Model file for the job. Use its own axes, mm. Give positions to 0.01 mm unless a question says otherwise; leave off trailing zeros. Loops run counter-clockwise (first coordinate to the right, second up) from the corner with the lowest first, then second, coordinate; pieces in that order, holes last. Notation, with made-up numbers: M 20.25,66.5 L 39.25,66.5 A7 ccw 39.25,79.5 Z; hole C -0.5,9 d5. An arc over 180 degrees is marked long. Use CSV: the item, a comma, the result in double quotes. Start each with the question number.
(1) Wall check: line 1 along X through (y, z) = (-0.05, 8.89) (3 decimals); line 2 along X through (y, z) = (2.5, 16.5); line 3 along Y through (x, z) = (-41.5, -7.5). Give the ranges that are in metal, low to high. Write a range as from..to.
(2) Slice it at A-A on x = 60.5. List the corners of the cut face in (y, z).
(3) Flat gauge pins, fed straight in: P1, Ø4, axis at x = 14.86, z = -7.65, coming from the -Y side; P2, Ø1.4, axis at y = 0.5, z = -6, coming from the +X side; P3, Ø3, axis at y = -0.5, z = 16, coming from the -X side; P4, Ø15, axis at x = -34.925, z = 8.89, coming from the -Y side. Where does each tip first touch, or does it go through?
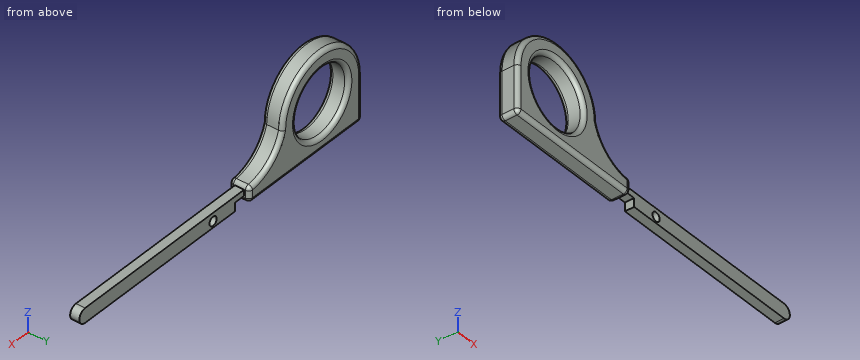
```python
from build123d import *

# Parameters (mm, degrees)
F0_R     = 12.7
F0_R_2   = 1.7145
F1_DEPTH = 1.778
F2_DEPTH = 3.81
F3_R     = 1.524


with BuildPart() as f1:
    # F0 (on Front) → F1 (new body, symmetric)
    with BuildSketch(Plane.XZ):
        with BuildLine():
            ThreePointArc((-15.875, 8.889999828), (-34.925, 27.939999828), (-53.975, 8.889999828))
            Line((-53.975, 8.889999828), (-53.975, -7.366000172))
            ThreePointArc((-53.975, -7.366000172), (-53.5286307345, -8.4436309065), (-52.451, -8.890000172))
            Line((-52.451, -8.890000172), (-1.5220896796, -8.890000172))
            ThreePointArc((-1.5220896796, -8.890000172), (-0.4444589451, -8.4436309065), (0.0019103204, -7.366000172))
            Line((0.0019103204, -7.366000172), (0.0019103204, -6.7696216721))
            Line((0.0019103204, -6.7696216721), (0.0019103204, -4.4836216721))
            ThreePointArc((0.0019103204, -4.4836216721), (-0.4004734297, -3.4520068765), (-1.3949844225, -2.9650883473))
            ThreePointArc((-1.3949844225, -2.9650883473), (-10.4768897023, 0.7127293809), (-15.875, 8.889999828))
        make_face()
        with Locations((-34.925, 8.889999828)):
            Circle(F0_R, mode=Mode.SUBTRACT)
        with BuildLine():
            Line((76.2019103204, -4.4836216721), (0.0019103204, -4.4836216721))
            Line((0.0019103204, -4.4836216721), (0.0019103204, -6.7696216721))
            Line((0.0019103204, -6.7696216721), (4.3199103204, -6.7696216721))
            Line((4.3199103204, -6.7696216721), (4.3199103204, -10.0716216721))
            Line((4.3199103204, -10.0716216721), (76.2019103204, -10.0716216721))
            ThreePointArc((76.2019103204, -10.0716216721), (78.9959103204, -7.2776216721), (76.2019103204, -4.4836216721))
        make_face()
        with Locations((14.8609103204, -7.6513164506)):
            Circle(F0_R_2, mode=Mode.SUBTRACT)
    extrude(amount=F1_DEPTH, both=True)

    # F0 (on Front) → F2 (join, symmetric)
    with BuildSketch(Plane.XZ):
        with BuildLine():
            ThreePointArc((-15.875, 8.889999828), (-34.925, 27.939999828), (-53.975, 8.889999828))
            Line((-53.975, 8.889999828), (-53.975, -7.366000172))
            ThreePointArc((-53.975, -7.366000172), (-53.5286307345, -8.4436309065), (-52.451, -8.890000172))
            Line((-52.451, -8.890000172), (-1.5220896796, -8.890000172))
            ThreePointArc((-1.5220896796, -8.890000172), (-0.4444589451, -8.4436309065), (0.0019103204, -7.366000172))
            Line((0.0019103204, -7.366000172), (0.0019103204, -6.7696216721))
            Line((0.0019103204, -6.7696216721), (0.0019103204, -4.4836216721))
            ThreePointArc((0.0019103204, -4.4836216721), (-0.4004734297, -3.4520068765), (-1.3949844225, -2.9650883473))
            ThreePointArc((-1.3949844225, -2.9650883473), (-10.4768897023, 0.7127293809), (-15.875, 8.889999828))
        make_face()
        with Locations((-34.925, 8.889999828)):
            Circle(F0_R, mode=Mode.SUBTRACT)
    extrude(amount=F2_DEPTH, both=True)

    # F3
    f3_edges = [f1.edges().sort_by_distance(p)[0] for p in [
        (-34.925, -3.81, 27.94),
        (-47.625, -3.81, 8.89),
        (-47.625, 3.81, 8.89),
        (-34.925, 3.81, 27.94),
    ]]
    fillet(f3_edges, radius=F3_R)


solid = f1.part
```
Reply:
1,line 1,"x = -53.975..-47.625, -22.225..-15.875"
1,line 2,"x = -52.37..-45.11, -24.74..-17.48"
1,line 3,"y = -3.8..3.8"
2,outline,"M -1.78,-10.07 L 1.78,-10.07 L 1.78,-4.48 L -1.78,-4.48 Z"
3,P1,"stops at y = -1.78"
3,P2,"stops at x = 78.94"
3,P3,"stops at x = -53.13"
3,P4,"passes through"
